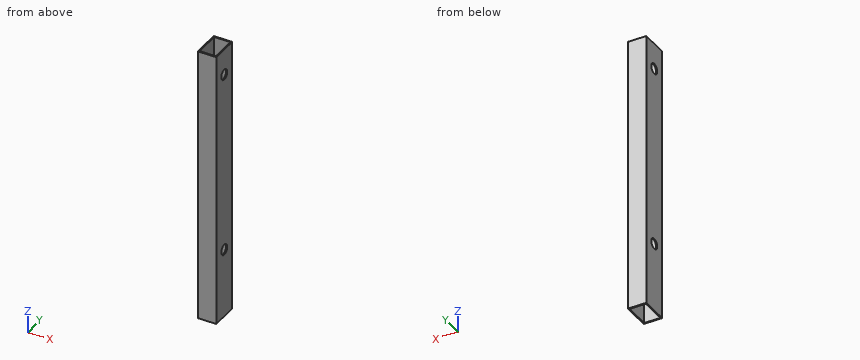
from build123d import *

# Parameters (mm, degrees)
SKETCH1_W           = 50.8
SKETCH1_H           = 76.2
SKETCH1_W_2         = 44.45
SKETCH1_H_2         = 69.85
BOSS_EXTRUDE1_DEPTH = 762
CUT_EXTRUDE1_REACH  = 766.641
SKETCH4_R           = 14.224


with BuildPart() as part:
    # Sketch1 → Boss-Extrude1 (new body)
    with BuildSketch(Plane.XY):
        Rectangle(SKETCH1_W, SKETCH1_H)
        Rectangle(SKETCH1_W_2, SKETCH1_H_2, mode=Mode.SUBTRACT)
    extrude(amount=BOSS_EXTRUDE1_DEPTH)

    # Cut-Extrude1: up to this face of the body (flat: up to its plane)
    cut_extrude1_end = Plane(part.part.faces().sort_by_distance((-25.4, 0, 381))[0])
    # Sketch4 → Cut-Extrude1 (cut, up to the picked face)
    with BuildSketch(Plane(origin=(25.4, 0, 0), x_dir=(0, 0, -1), z_dir=(1, 0, 0)), mode=Mode.PRIVATE) as cut_extrude1_sk1:
        with Locations(Location((-690.548048411, 0, 0), (0, 0, 90))):
            Circle(SKETCH4_R)
    cut_extrude1_tool1 = split(extrude(cut_extrude1_sk1.sketch, amount=-CUT_EXTRUDE1_REACH, mode=Mode.PRIVATE), bisect_by=cut_extrude1_end, keep=Keep.BOTH, mode=Mode.PRIVATE)
    # Sketch4 → Cut-Extrude1 (cut, up to the picked face)
    with BuildSketch(Plane(origin=(25.4, 0, 0), x_dir=(0, 0, -1), z_dir=(1, 0, 0)), mode=Mode.PRIVATE) as cut_extrude1_sk2:
        with Locations(Location((-190.549048411, 0, 0), (0, 0, 90))):
            Circle(SKETCH4_R)
    cut_extrude1_tool2 = split(extrude(cut_extrude1_sk2.sketch, amount=-CUT_EXTRUDE1_REACH, mode=Mode.PRIVATE), bisect_by=cut_extrude1_end, keep=Keep.BOTH, mode=Mode.PRIVATE)
    add(cut_extrude1_tool1.solids().sort_by(Axis((25.4, 0, 690.548048), (-1, 0, 0)))[0], mode=Mode.SUBTRACT)
    add(cut_extrude1_tool2.solids().sort_by(Axis((25.4, 0, 190.549048), (-1, 0, 0)))[0], mode=Mode.SUBTRACT)


solid = part.part
The model under review builds one solid part; all positions refer to its coordinate system, in mm. Round coordinates to 2 decimals unless told otherwise and drop trailing zeros. Loops run counter-clockwise (first coordinate to the right, second up) from the corner with the lowest first, then second, coordinate; pieces in that order, holes last. Notation, with made-up numbers: M -39.75,79 L 10.25,79 A30 ccw 10.25,116 Z; hole C 48.25,78.25 d11. An arc over 180 degrees is marked long. Answer as a JSON object with one key per item and string values.
Item 1: We need section A-A, the plane x = -12. State the section outline as (y, z) points (3 decimals), and give its area (3 significant figures).
Check sheet entries:
{"outline": "M -38.1,0 L -34.925,0 L -34.925,762 L -38.1,762 Z; M 34.925,0 L 38.1,0 L 38.1,762 L 34.925,762 Z", "area": "4,840 mm2"}
Item 2: We need section C-C, the plane z = 421. State the section outline as (x, y) points (3 decimals).
Check sheet entries:
{"outline": "M -25.4,-38.1 L 25.4,-38.1 L 25.4,38.1 L -25.4,38.1 Z; hole M -22.225,-34.925 L 22.225,-34.925 L 22.225,34.925 L -22.225,34.925 Z"}
Item 3: For line 1 along Z through (x, y) = (23, 0); line 2 along X through (y, z) = (-20, 680.5) (3 decimals); line 3 along Y through (x, z) = (9.5, 294.5) (3 decimals), list the stretches that pass through material, from the lowest coordinate up.
Check sheet entries:
{"line 1": "0 to 176.33, 204.77 to 676.32, 704.77 to 762", "line 2": "-25.4 to -22.225, 22.225 to 25.4", "line 3": "-38.1 to -34.925, 34.925 to 38.1"}
Item 4: We need section B-B, the plane y = -23.5. State the section outline as (x, z) points (3 decimals), and give its area (3 significant figures).
Check sheet entries:
{"outline": "M -25.4,0 L -22.225,0 L -22.225,762 L -25.4,762 Z; M 22.225,0 L 25.4,0 L 25.4,762 L 22.225,762 Z", "area": "4,840 mm2"}
